The figure shows three views and two pictorial views of one solid part (mm, origin at its lowest corner). Answer the questions. A direction names the side the tool comes from. Coordinates: 2 decimals unless noted, no trailing zeros. Order: outer loops, then holes, each group sorted by start corner. A loop starts at its lowest first (then second) coordinate and runs counter-clockwise, first axis right, second up. Notation, with made-up numbers: M -27,9 L 13,9 A25 cw 13,33 Z; hole C 71.25,38 d1. An arc over 180 degrees is marked long. Answer in a Markdown table with one row per item. Add a question column.
Item 1: The part is cut by section C-C (z = 1.5). Write down the section's boundary in (x, y), then the cut area to 3 significant figures.
Item 2: The part is cut by section D-D (y = 23). Write down the section's boundary in (x, z).
Item 3: Which of the six approach directions +Z, -Z, +X, -X, +Y, -Y give full straight-line access (tool end or side, diameter ignored) to the marked faces 1 and 2?
Item 4: Flat-ended cylindrical pins translate along their axes: pin 1 Ø6 at (y, z) = (5.5, 4.5) entering from +X; pin 2 Ø1.5 at (x, z) = (12, 8.5) entering from +Y; pin 3 Ø15.5 at (x, y) = (16, 16) entering from +Z. Find the tip coordinate at first contact, or state that the pin passes through.
Item 5: The part is cut by section A-A (y = 16). Write down the section's boundary in (x, z).
Item 6: Consider line 1 (Y direction, x = 16, z = 8); line 2 (Y direction, x = 16, z = 0.45); line 3 (X direction, y = 19.5, z = 7.5). Determine where each line is inside the solid, lowest interval first. Write a range as from..to.
Item 7: The mould has two halves that part along X. Classify the marked faces 3, 4, 5 and 6: released by +X, released by -X, zero draft, split by the parting line, or undercut.
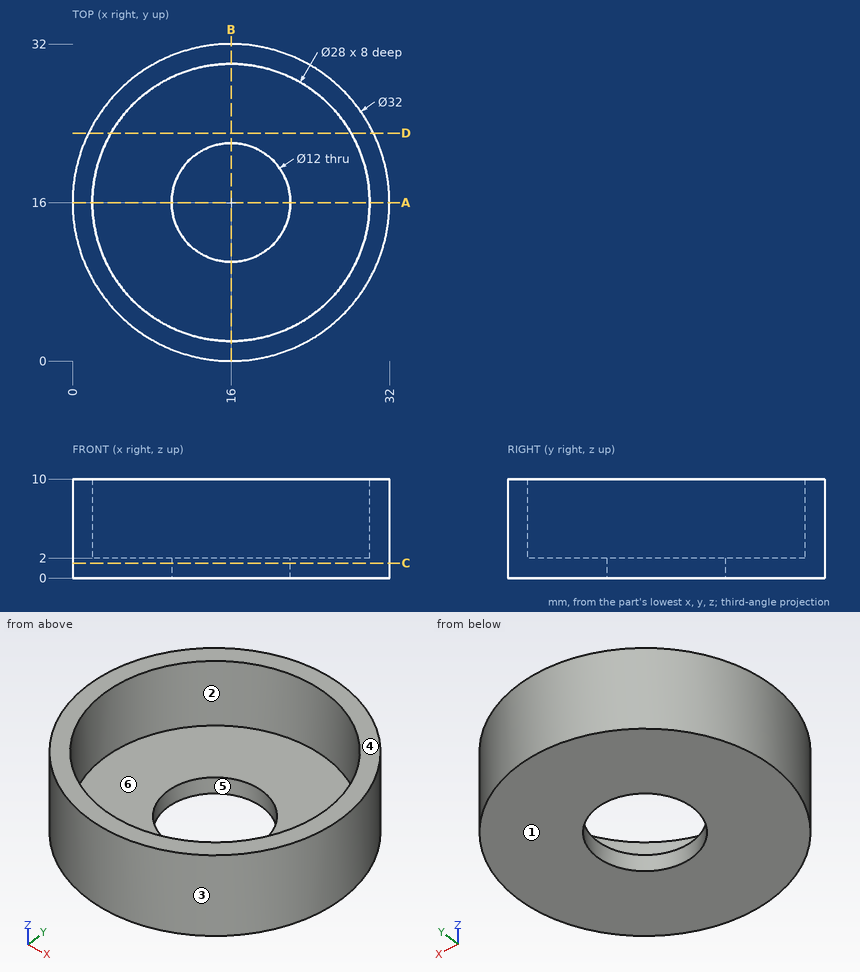
Reply:
| question | item | result |
|---|---|---|
| 1 | outline | C 16,16 d32; hole C 16,16 d12 |
| 1 | area | 691 mm2 |
| 2 | outline | M 1.61,0 L 30.39,0 L 30.39,10 L 28.12,10 L 28.12,2 L 3.88,2 L 3.88,10 L 1.61,10 Z |
| 3 | face 1 | -Z, +X, -X, +Y, -Y |
| 3 | face 2 | +Z |
| 4 | pin 1 | stops at x = 30.13 |
| 4 | pin 2 | stops at y = 31.67 |
| 4 | pin 3 | stops at z = 2 |
| 5 | outline | M 0,0 L 10,0 L 10,2 L 2,2 L 2,10 L 0,10 Z; M 22,0 L 32,0 L 32,10 L 30,10 L 30,2 L 22,2 Z |
| 6 | line 1 | y = 0..2, 30..32 |
| 6 | line 2 | y = 0..10, 22..32 |
| 6 | line 3 | x = 0.39..2.44, 29.56..31.61 |
| 7 | face 3 | split by the parting line |
| 7 | face 4 | zero draft |
| 7 | face 5 | undercut |
| 7 | face 6 | undercut |
